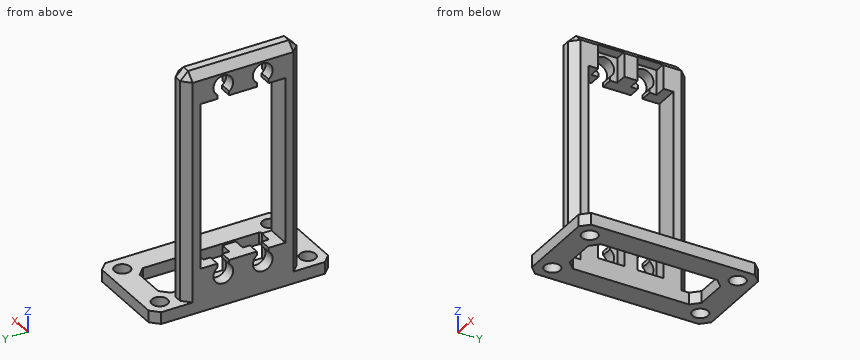
```python
from build123d import *

# Parameters (mm, degrees)
SKETCH1_W           = 58
SKETCH1_H           = 29.5
BOSS_EXTRUDE1_DEPTH = 6
SKETCH2_W           = 6.6
SKETCH2_H           = 6.6
CUT_EXTRUDE1_DEPTH  = 3
SKETCH3_W           = 24
SKETCH3_H           = 45.5
SKETCH3_R           = 2
SKETCH3_W_2         = 12
SKETCH3_H_2         = 33.5
BOSS_EXTRUDE2_DEPTH = 3
CHAMFER5_SIZE       = 2
CHAMFER6_SIZE       = 2
CHAMFER7_SIZE       = 2


with BuildPart() as part:
    # Sketch1 → Boss-Extrude1 (new body)
    with BuildSketch(Plane(origin=(0, 0, 0), x_dir=(0, 0, -1), z_dir=(1, 0, 0))):
        with Locations((-9.508456449, 0.450525737)):
            Rectangle(SKETCH1_W, SKETCH1_H)
        with BuildLine():
            Line((-31.508456449, 6.950525737), (-30.508456449, 6.950525737))
            Line((-30.508456449, 6.950525737), (-30.508456449, 11.200525737))
            Line((-30.508456449, 11.200525737), (11.491543551, 11.200525737))
            Line((11.491543551, 11.200525737), (11.491543551, 6.950525737))
            Line((11.491543551, 6.950525737), (12.491543551, 6.950525737))
            ThreePointArc((12.491543551, 6.950525737), (16.991543551, 5.450525737), (12.491543551, 3.950525737))
            Line((12.491543551, 3.950525737), (11.491543551, 3.950525737))
            Line((11.491543551, 3.950525737), (11.491543551, -3.049474263))
            Line((11.491543551, -3.049474263), (12.491543551, -3.049474263))
            ThreePointArc((12.491543551, -3.049474263), (16.991543551, -4.549474263), (12.491543551, -6.049474263))
            Line((12.491543551, -6.049474263), (11.491543551, -6.049474263))
            Line((11.491543551, -6.049474263), (11.491543551, -10.299474263))
            Line((11.491543551, -10.299474263), (-30.508456449, -10.299474263))
            Line((-30.508456449, -10.299474263), (-30.508456449, -6.049474263))
            Line((-30.508456449, -6.049474263), (-31.508456449, -6.049474263))
            ThreePointArc((-31.508456449, -6.049474263), (-36.008456449, -4.549474263), (-31.508456449, -3.049474263))
            Line((-31.508456449, -3.049474263), (-30.508456449, -3.049474263))
            Line((-30.508456449, -3.049474263), (-30.508456449, 3.950525737))
            Line((-30.508456449, 3.950525737), (-31.508456449, 3.950525737))
            ThreePointArc((-31.508456449, 3.950525737), (-36.008456449, 5.450525737), (-31.508456449, 6.950525737))
        make_face(mode=Mode.SUBTRACT)
    extrude(amount=BOSS_EXTRUDE1_DEPTH)

    # Sketch2 → Cut-Extrude1 (cut)
    with BuildSketch(Plane(origin=(6, 0, 0), x_dir=(0, 0, -1), z_dir=(1, 0, 0))):
        with Locations((-33.508456449, 5.450525737)):
            Rectangle(SKETCH2_W, SKETCH2_H)
        with Locations((14.491543551, 5.450525737)):
            Rectangle(SKETCH2_W, SKETCH2_H)
        with Locations((-33.508456449, -4.549474263)):
            Rectangle(SKETCH2_W, SKETCH2_H)
        with Locations((14.491543551, -4.549474263)):
            Rectangle(SKETCH2_W, SKETCH2_H)
    extrude(amount=-CUT_EXTRUDE1_DEPTH, mode=Mode.SUBTRACT)

    # Sketch3 → Boss-Extrude2 (add)
    with BuildSketch(Plane(origin=(0, 0, -19.491543551), x_dir=(-1, 0, 0), z_dir=(0, 0, -1))):
        with Locations((-12, 0.450525737)):
            Rectangle(SKETCH3_W, SKETCH3_H)
        with Locations(Location((-4, 19.200525737, 0), (0, 0, 90))):
            Circle(SKETCH3_R, mode=Mode.SUBTRACT)
        with Locations(Location((-20, 19.200525737, 0), (0, 0, 270))):
            Circle(SKETCH3_R, mode=Mode.SUBTRACT)
        with Locations(Location((-20, -18.299474263, 0), (0, 0, 90))):
            Circle(SKETCH3_R, mode=Mode.SUBTRACT)
        with Locations(Location((-4, -18.299474263, 0), (0, 0, 270))):
            Circle(SKETCH3_R, mode=Mode.SUBTRACT)
        with Locations((-12, 0.450525737)):
            Rectangle(SKETCH3_W_2, SKETCH3_H_2, mode=Mode.SUBTRACT)
    extrude(amount=BOSS_EXTRUDE2_DEPTH)

    # Chamfer5
    chamfer5_edges = [part.edges().sort_by_distance(p)[0] for p in [
        (6, 17.200525737, -20.991543551),
        (18, 17.200525737, -20.991543551),
        (18, -16.299474263, -20.991543551),
        (6, -16.299474263, -20.991543551),
    ]]
    chamfer(chamfer5_edges, length=CHAMFER5_SIZE)

    # Chamfer6
    chamfer6_edges = [part.edges().sort_by_distance(p)[0] for p in [
        (24, -22.299474263, -20.991543551),
        (0, -22.299474263, -20.991543551),
        (0, 23.200525737, -20.991543551),
        (24, 23.200525737, -20.991543551),
    ]]
    chamfer(chamfer6_edges, length=CHAMFER6_SIZE)

    # Chamfer7
    # the kernel refuses this chamfer: 2 mm, written as the material it takes off along each edge
    with BuildSketch(Plane(origin=(4.666666667, 13.867192404, 37.175123115), x_dir=(0.7071067811865474, -0.7071067811865477, 0), z_dir=(0.577350269189626, 0.5773502691896257, 0.5773502691896257)), Plane(origin=(1.333333333, 13.867192404, 37.175123115), x_dir=(0.7071067811865477, 0.7071067811865474, 0), z_dir=(-0.5773502691896256, 0.5773502691896258, 0.5773502691896258))) as chamfer7_piece_1:
        Polygon((-1.414213562, 0.816496581), (1.414213562, 0.816496581), (0, -1.632993162), align=None)
    extrude(amount=2.540341184, mode=Mode.SUBTRACT)
    with BuildSketch(Plane(origin=(4.666666667, -12.966140929, 37.175123115), x_dir=(0.7071067811865474, 0.7071067811865477, 0), z_dir=(0.577350269189626, -0.5773502691896257, 0.5773502691896257)), Plane(origin=(1.333333333, -12.966140929, 37.175123115), x_dir=(0.7071067811865477, -0.7071067811865474, 0), z_dir=(-0.5773502691896256, -0.5773502691896258, 0.5773502691896258))) as chamfer7_piece_2:
        Polygon((-1.414213562, -0.816496581), (1.414213562, -0.816496581), (0, 1.632993162), align=None)
    extrude(amount=2.540341184, mode=Mode.SUBTRACT)
    with BuildSketch(Plane(origin=(6, 15.200525737, 43.651822425), x_dir=(-0.9996219169112968, 0.027495876610586494, 0), z_dir=(0, 0, -1)), Plane(origin=(6, -14.299474263, -19.491543551), x_dir=(-0.9996219169112968, -0.027495876610586494, 0), z_dir=(0, 0, 1)), Plane(origin=(0, -14.299474263, -19.491543551), x_dir=(-0.027495876610586795, 0.9996219169112968, 0), z_dir=(0, 0, 1)), Plane(origin=(0, 15.200525737, 43.651822425), x_dir=(-0.027495876610586365, -0.9996219169112968, 0), z_dir=(0, 0, -1))) as chamfer7_piece_3:
        Polygon((CHAMFER7_SIZE * 0.999621916911, -CHAMFER7_SIZE * 0.0274958766106), (-CHAMFER7_SIZE * 0.0274958766106, -CHAMFER7_SIZE * 0.999621916911), (0, 0), align=None)
    extrude(amount=63.143365976, mode=Mode.SUBTRACT)
    with BuildSketch(Plane(origin=(6, -19.442840238, 38.508456449), x_dir=(-0.9996219169112968, 0, 0.02749587661058563), z_dir=(0, 1, 0)), Plane(origin=(0, -19.442840238, 38.508456449), x_dir=(-0.02749587661058639, 0, -0.9996219169112968), z_dir=(0, 1, 0))) as chamfer7_piece_4:
        Polygon((CHAMFER7_SIZE * 0.999621916911, -CHAMFER7_SIZE * 0.0274958766106), (-CHAMFER7_SIZE * 0.0274958766106, -CHAMFER7_SIZE * 0.999621916911), (0, 0), align=None)
    extrude(amount=39.786731952, mode=Mode.SUBTRACT)
    with BuildSketch(Plane(origin=(-5.143365976, -14.299474263, 38.508456449), x_dir=(0, -0.02749587661058651, -0.9996219169112968), z_dir=(1, 0, 0))) as chamfer7_piece_5:
        Polygon((CHAMFER7_SIZE * 0.999621916911, CHAMFER7_SIZE * 0.0274958766106), (-CHAMFER7_SIZE * 0.0274958766106, CHAMFER7_SIZE * 0.999621916911), (0, 0), align=None)
    extrude(amount=16.286731952, mode=Mode.SUBTRACT)
    with BuildSketch(Plane(origin=(-5.143365976, 15.200525737, 38.508456449), x_dir=(0, 0.02749587661058651, -0.9996219169112968), z_dir=(1, 0, 0))) as chamfer7_piece_6:
        Polygon((CHAMFER7_SIZE * 0.999621916911, -CHAMFER7_SIZE * 0.0274958766106), (-CHAMFER7_SIZE * 0.0274958766106, -CHAMFER7_SIZE * 0.999621916911), (0, 0), align=None)
    extrude(amount=16.286731952, mode=Mode.SUBTRACT)


solid = part.part
```
Build history of the part. All positions in model axes, mm. Round coordinates to 2 decimals unless told otherwise and drop trailing zeros. Loops run counter-clockwise (first coordinate to the right, second up) from the corner with the lowest first, then second, coordinate; pieces in that order, holes last.
Item 1: Saw through at C-C (z = 6.5). List the corners of the cut face in (x, y).
Item 2: Drill centre lines: line 1 along Y through (x, z) = (4.5, 31.5); line 2 along Y through (x, z) = (2, -15); line 3 along X through (y, z) = (11.5, 35). Where is each one in solid material? Low to high.
Item 3: Saw through at D-D (z = 33.5). List the corners of the cut face in (x, y).
Item 4: Saw through at B-B (x = 20). List the corners of the cut face in (y, z).
Item 5: Saw through at A-A (x = 14.75). List the corners of the cut face in (y, z).
Item 6: Pin check, flat tips, straight feed: P1, Ø3.5, axis at x = 5, z = 33, coming from the +Y side; P2, Ø0.9, axis at x = 5, z = -14, coming from the +Y side; P3, Ø6, axis at y = -8, z = 26, coming from the +X side; P4, Ø4.5, axis at x = 20, y = -18.3, coming from the -Z side. Stop position of each tip, or through.
Worked answers:
1. outline: (0, -12.3) - (2, -14.3) - (4, -14.3) - (6, -12.3) - (6, -10.3) - (0, -10.3) - close; (0, 11.2) - (6, 11.2) - (6, 13.2) - (4, 15.2) - (2, 15.2) - (0, 13.2) - close
2. line 1: y = -13.8 to -7.85, -1.25 to 2.15, 8.75 to 14.7
2. line 2: y = -14.3 to -7, -2.1 to 3, 7.9 to 15.2
2. line 3: x = 0 to 6
3. outline: (0, -12.3) - (2, -14.3) - (4, -14.3) - (6, -12.3) - (6, -7.85) - (3, -7.85) - (3, -7.05) - (0, -7.05) - close; (0, -2.05) - (3, -2.05) - (3, -1.25) - (6, -1.25) - (6, 2.15) - (3, 2.15) - (3, 2.95) - (0, 2.95) - close; (0, 7.95) - (3, 7.95) - (3, 8.75) - (6, 8.75) - (6, 13.2) - (4, 15.2) - (2, 15.2) - (0, 13.2) - close
4. outline: (-22.3, -22.49) - (-20.3, -22.49) - (-20.3, -19.49) - (-22.3, -19.49) - close; (-16.3, -22.49) - (17.2, -22.49) - (17.2, -19.49) - (-16.3, -19.49) - close; (21.2, -22.49) - (23.2, -22.49) - (23.2, -19.49) - (21.2, -19.49) - close
5. outline: (-22.3, -22.49) - (-16.3, -22.49) - (-16.3, -19.49) - (-22.3, -19.49) - close; (17.2, -22.49) - (23.2, -22.49) - (23.2, -19.49) - (17.2, -19.49) - close
6. P1: stops at y = 15.2
6. P2: stops at y = 14.65
6. P3: stops at x = 6
6. P4: stops at z = -22.49
